Could you check a few things on this model? Use its own coordinates, in mm. Round coordinates to 2 decimals unless told otherwise and drop trailing zeros. Write each loop counter-clockwise with the first axis right and the second up, starting at its lowest first coordinate (ties: lowest second). Pieces come first, ordered by that corner, then holes. Notation, with made-up numbers: (-25.75, 33) -> (-15.75, 33) arc R4 cw to (-15.75, 39) -> close; hole circle Ø8 at (88, 5). An arc over 180 degrees is marked (long way). Return JSON: item names as keys, results as strings.
Autodesk Inventor part; units mm, degrees
ref_plane "YZ Plane" through (0, 0, 0) normal (1, 0, 0) x (0, 1, 0)
ref_plane "XZ Plane" through (0, 0, 0) normal (0, 1, 0) x (-1, 0, 0)
ref_plane "XY Plane" through (0, 0, 0) normal (0, 0, 1) x (1, 0, 0)
sketch "Sketch1" plane through (0, 0, 0) normal (1, 0, 0) x (0, 1, 0)
  line L0 (0, 0) -> (400, 0)
  line L1 (400, 0) -> (400, -350)
  line L2 (400, -350) -> (0, -350)
  line L3 (0, -350) -> (0, 0)
  dimension "d0" = 400
  dimension "d1" = 350
extrude "Extrusion1" add sketch "Sketch1" along normal blind 0.607
sketch "Sketch2" plane through (0.607, 0, 0) normal (1, 0, 0) x (0, 0, -1)
  line L0 (0, 399.8291) -> (174.9999, 400)
  line L1 (350, 400) -> (0, 400)
  line L2 (174.9999, 400) -> (175.0243, 375)
  circle A0 centre (175.0243, 375) radius 7.5
  line L3 (175.0243, 375) -> (87.5243, 375)
  line L4 (175.0243, 375) -> (262.5243, 375)
  circle A1 centre (87.5243, 375) radius 7.5
  circle A2 centre (262.5243, 375) radius 7.5
  point P0 (0, 0)
  dimension "d4" = 175
  dimension "d5" = 25
  dimension "d7" = 15
  dimension "d12" = 15
  dimension "d13" = 15
extrude "Extrusion2" cut sketch "Sketch2" against normal through all
equation "\"BendRadius\" = Thickness"
equation "\"BendReliefWidth\" = Thickness"
equation "\"BendReliefDepth\" = 0.5 * Thickness"
equation "\"CornerReliefSize\" = 4 * Thickness"
equation "\"MinimumRemnant\" = 2 * Thickness"
equation "\"TransitionRadius\" = BendRadius"
equation "\"JacobiRadiusSize\" = BendRadius"
equation "\"GapSize\" = Thickness"
properties part number "project Backrestfinal" material "Steel, Galvanized"
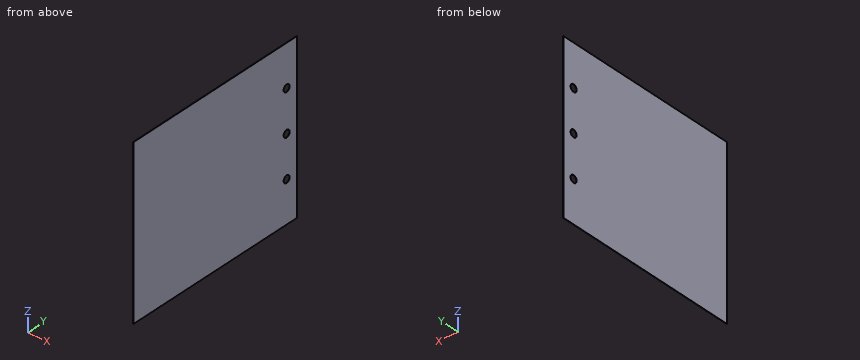
1) If I drill on probe 1 along Z at (x, y) = (0.2, 375); probe 2 along Y at (x, z) = (0.4, -264.5); probe 3 along Y at (x, z) = (0.4, -171.5), over which ranges is the centre line in solid material (lowest first)? Write a range as [from, to].
Return value:
{"probe 1": "[-350, -270.02], [-255.02, -182.52], [-167.52, -95.02], [-80.02, 0]", "probe 2": "[0, 367.76], [382.24, 400]", "probe 3": "[0, 368.38], [381.62, 400]"}
2) I want a section at A-A, the plane y = 375. Please give me the cut outline in (x, z).
Return value:
{"outline": "(0, -350) -> (0.61, -350) -> (0.61, -270.02) -> (0, -270.02) -> close; (0, -255.02) -> (0.61, -255.02) -> (0.61, -182.52) -> (0, -182.52) -> close; (0, -167.52) -> (0.61, -167.52) -> (0.61, -95.02) -> (0, -95.02) -> close; (0, -80.02) -> (0.61, -80.02) -> (0.61, 0) -> (0, 0) -> close"}
3) Will this pin go through, and if not, where does the flat tip stop? pin 1 Ø12 at (y, z) = (375, -262.52) entering from +X.
Return value:
{"pin 1": "through"}
